Read the model definition and answer for the solid it produces. Units are mm, in the model's axes. Coordinates: 2 decimals unless noted, no trailing zeros. Order: outer loops, then holes, each group sorted by start corner. A loop starts at its lowest first (then second) coordinate and runs counter-clockwise, first axis right, second up.
```python
from build123d import *

# Parameters (mm, degrees)
SKETCH1_R          = 8
EXTRUDE1_DEPTH     = 946
SKETCH3_R          = 8
SKETCH3_R_2        = 6
CUT_EXTRUDE1_DEPTH = 54
SKETCH4_R          = 8
SKETCH4_R_2        = 6
CUT_EXTRUDE2_DEPTH = 20
SKETCH5_R          = 8
SKETCH5_R_2        = 6
EXTRUDE2_DEPTH     = 3
SKETCH6_R          = 8
SKETCH6_R_2        = 6
EXTRUDE3_DEPTH     = 3


with BuildPart() as part:
    # Sketch1 → Extrude1 (new body)
    with BuildSketch(Plane.XY):
        Circle(SKETCH1_R)
    extrude(amount=EXTRUDE1_DEPTH)

    # Sketch3 → Cut-Extrude1 (cut)
    with BuildSketch(Plane.XY.offset(946)):
        Circle(SKETCH3_R)
        Circle(SKETCH3_R_2, mode=Mode.SUBTRACT)
    extrude(amount=-CUT_EXTRUDE1_DEPTH, mode=Mode.SUBTRACT)

    # Sketch4 → Cut-Extrude2 (cut)
    with BuildSketch(Plane(origin=(0, 0, 0), x_dir=(-1, 0, 0), z_dir=(0, 0, -1))):
        Circle(SKETCH4_R)
        Circle(SKETCH4_R_2, mode=Mode.SUBTRACT)
    extrude(amount=-CUT_EXTRUDE2_DEPTH, mode=Mode.SUBTRACT)

    # Sketch5 → Extrude2 (add)
    with BuildSketch(Plane(origin=(0, 0, 20), x_dir=(-1, 0, 0), z_dir=(0, 0, -1))):
        Circle(SKETCH5_R)
        Circle(SKETCH5_R_2, mode=Mode.SUBTRACT)
    extrude(amount=EXTRUDE2_DEPTH)

    # Sketch6 → Extrude3 (add)
    with BuildSketch(Plane.XY.offset(892)):
        Circle(SKETCH6_R)
        Circle(SKETCH6_R_2, mode=Mode.SUBTRACT)
    extrude(amount=EXTRUDE3_DEPTH)


solid = part.part
```
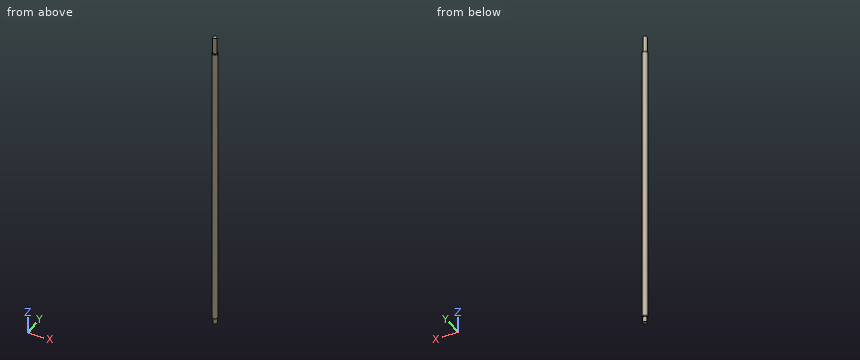
1) Straight lines are drawn through the part: line 1 (Z direction, x = -5, y = -6); line 2 (X direction, y = -0.75, z = 154); line 3 (Y direction, x = 1.5, z = 373). For each, find the intervals that lie inside material, in ascending order.
A:
line 1: z = 17 to 895
line 2: x = -7.96 to 7.96
line 3: y = -7.86 to 7.86
2) A cutting plane is placed at A-A, the plane x = 0. Determine the outline of the cut face in (y, z).
A:
outline: (-8, 17) - (-6, 17) - (-6, 0) - (6, 0) - (6, 17) - (8, 17) - (8, 895) - (6, 895) - (6, 946) - (-6, 946) - (-6, 895) - (-8, 895) - close
3) A cutting plane is placed at C-C, the plane z = 391. Determine the outline of the cut face in (x, y).
A:
outline: circle Ø16 at (0, 0)
4) Flat-ended cylindrical pins translate along their axes: pin 1 Ø4 at (y, z) = (4.5, 388) entering from +X; pin 2 Ø4 at (y, z) = (-2.5, 596) entering from +X; pin 3 Ø2 at (y, z) = (-4.5, 547.5) entering from -X. Find the tip coordinate at first contact, or state that the pin passes through.
A:
pin 1: stops at x = 7.6
pin 2: stops at x = 7.98
pin 3: stops at x = -7.19
